CAD build for the part. Positions are in the model's coordinates, mm. Coordinates: 2 decimals unless noted, no trailing zeros. Loops run counter-clockwise (first coordinate to the right, second up) from the corner with the lowest first, then second, coordinate; pieces in that order, holes last.
1) Saw through at A-A, the plane y = 8. Write the cut outline in (x, z).
2) Saw through at C-C, the plane x = -45.5. Write the cut outline in (y, z).
3) Saw through at D-D, the plane y = 11.5. Write the cut outline in (x, z).
4) Saw through at B-B, the plane z = 1.7. Write the cut outline in (x, y), and give its area (3 significant figures).
5) Pin check, flat tips, straight feed: pin 1 Ø1 at (y, z) = (20, 1.5) entering from -X; pin 2 Ø1 at (x, z) = (-54.5, 2) entering from +Y. Stop position of each tip, or through.
6) Wall check: line 1 along X through (y, z) = (6.5, 1.7); line 2 along Y through (x, z) = (-62, 2.3); line 3 along X through (y, z) = (7.5, 1.95). Give the ranges that are in metal, low to high.
```python
from build123d import *

# Parameters (mm, degrees)
BOSS_EXTRUDE2_DEPTH = 2.54


with BuildPart() as part:
    # Sketch1 → Boss-Extrude2 (new body)
    with BuildSketch(Plane.XY):
        with BuildLine():
            Line((-48.545691329, 22.127640633), (-64.643124973, 10.698462746))
            Line((-64.643124973, 10.698462746), (-63.172663299, 8.627389965))
            ThreePointArc((-63.172663299, 8.627389965), (-62.225084369, 8.843975089), (-61.401896071, 8.327084411))
            Line((-61.401896071, 8.327084411), (-46.339998817, 19.021031462))
            Line((-46.339998817, 19.021031462), (-48.545691329, 22.127640633))
        make_face()
        with BuildLine():
            Line((-44.134306305, 15.914422291), (-46.339998817, 19.021031462))
            Line((-46.339998817, 19.021031462), (-61.401896071, 8.327084411))
            ThreePointArc((-61.401896071, 8.327084411), (-61.227467335, 7.977708977), (-61.167432462, 7.591853574))
            ThreePointArc((-61.167432462, 7.591853574), (-61.309016943, 7.00912), (-61.702201624, 6.556317184))
            Line((-61.702201624, 6.556317184), (-60.23173995, 4.485244403))
            Line((-60.23173995, 4.485244403), (-44.134306305, 15.914422291))
        make_face()
        with BuildLine():
            Line((-63.472968852, 6.856622737), (-65.60097568, 5.345737889))
            Line((-65.60097568, 5.345737889), (-63.395283168, 2.239128718))
            Line((-63.395283168, 2.239128718), (-60.23173995, 4.485244403))
            Line((-60.23173995, 4.485244403), (-61.702201624, 6.556317184))
            ThreePointArc((-61.702201624, 6.556317184), (-62.649780555, 6.33973206), (-63.472968852, 6.856622737))
        make_face()
        with BuildLine():
            Line((-64.643124973, 10.698462746), (-67.806668191, 8.452347061))
            Line((-67.806668191, 8.452347061), (-65.60097568, 5.345737889))
            Line((-65.60097568, 5.345737889), (-63.472968852, 6.856622737))
            ThreePointArc((-63.472968852, 6.856622737), (-63.689553976, 7.804201667), (-63.172663299, 8.627389965))
            Line((-63.172663299, 8.627389965), (-64.643124973, 10.698462746))
        make_face()
    extrude(amount=BOSS_EXTRUDE2_DEPTH)


solid = part.part
```
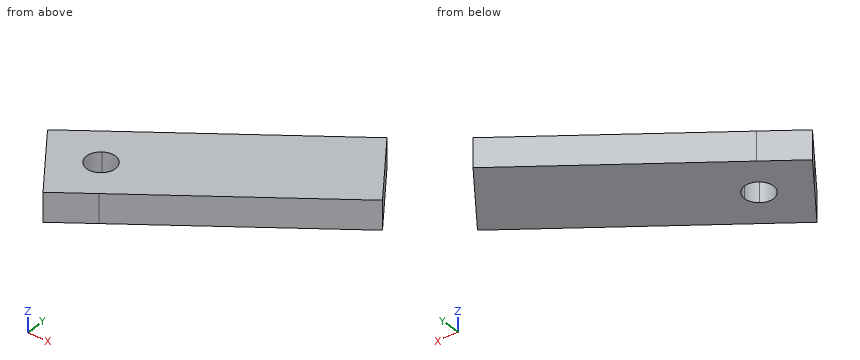
Data:
1. outline: (-67.49, 0) - (-63.64, 0) - (-63.64, 2.54) - (-67.49, 2.54) - close; (-61.23, 0) - (-55.28, 0) - (-55.28, 2.54) - (-61.23, 2.54) - close
2. outline: (14.94, 0) - (17.84, 0) - (17.84, 2.54) - (14.94, 2.54) - close
3. outline: (-63.51, 0) - (-50.35, 0) - (-50.35, 2.54) - (-63.51, 2.54) - close
4. outline: (-67.81, 8.45) - (-63.4, 2.24) - (-44.13, 15.91) - (-48.55, 22.13) - close; hole circle Ø2.54 at (-62.44, 7.59)
4. area: 175 mm2
5. pin 1: stops at x = -52.25
5. pin 2: stops at y = 18.26
6. line 1: x = -66.42 to -63.09, -61.79 to -57.39
6. line 2: y = 3.23 to 6.4, 8.78 to 12.58
6. line 3: x = -67.13 to -63.7, -61.17 to -55.99
